Check sheet for the modelled part. Datum: model origin and axes. Units: mm. Face numbers are marked on the shaded views. Round coordinates to 2 decimals unless told otherwise and drop trailing zeros. Order: outer loops, then holes, each group sorted by start corner. A loop starts at its lowest first (then second) coordinate and runs counter-clockwise, first axis right, second up.
(1) Mould release check, pull along X, two halves, no side actions. Record for the marked faces 1, 2, 3 and 4: released by +X, released by -X, zero draft, split by the parting line, or undercut.
(2) Depth check by flat-ended pin: pin 1 (3.5 mm diameter, centred on x = 5, y = 1, fed in from -Z); pin 2 (1.5 mm diameter, centred on x = 44.5, y = -14, fed in from +Z); pin 3 (1 mm diameter, centred on x = -36, z = -36.5, fed in from -Y); pin 4 (3 mm diameter, centred on x = 0, z = -6.25, fed in from +Y). Enter the tip coordinate at first touch or a pass-through.
(3) Sectioned sample at A-A, the plane x = -4. Enter the section's corners in (y, z), and give its area (3 significant figures).
(4) Sectioned sample at C-C, the plane y = -15. Enter the section's corners in (x, z).
(5) Thickness scan on probe 1 along Z at (x, y) = (-7.5, 1.25); probe 2 along X at (y, z) = (0.65, -6.25); probe 3 along Y at (x, z) = (-42.5, -26). Record the ranges inside material, lowest first.
(6) Sectioned sample at B-B, the plane y = -5.25. Enter the section's corners in (x, z), and give its area (3 significant figures).
```python
from build123d import *

# Parameters (mm, degrees)
BOSS_EXTRUDE1_DEPTH             = 2
BOSS_EXTRUDE2_DEPTH             = 17
BOSS_EXTRUDE2_DIRECTION_2_REACH = 86.623
SKETCH7_R                       = 4
CUT_EXTRUDE4_DEPTH              = 117.637747494
FILLET1_R                       = 1
CUT_EXTRUDE1_DEPTH              = 115.868304979
CUT_EXTRUDE2_DEPTH              = 89.209557156
SKETCH5_R                       = 2
CUT_EXTRUDE3_DEPTH              = 89.209557156


with BuildPart() as part:
    # Sketch1 → Boss-Extrude1 (new body)
    with BuildSketch(Plane(origin=(0, 0, 0), x_dir=(1, 0, 0), z_dir=(0, 1, 0))):
        Polygon((25, 46), (-25, 46), (-71, 0), (71, 0), align=None)
    extrude(amount=BOSS_EXTRUDE1_DEPTH)

    # Sketch2 → Boss-Extrude2 (add)
    with BuildSketch(Plane(origin=(0, 0, 0), x_dir=(-1, 0, 0), z_dir=(0, -1, 0))):
        Polygon((25, 46), (71, 0), (72.414213562, 1.414213562), (26.414213562, 47.414213562), align=None)
        Polygon((-26.414213562, 47.414213562), (-72.414213562, 1.414213562), (-71, 0), (-25, 46), align=None)
    extrude(amount=BOSS_EXTRUDE2_DEPTH)

    # Boss-Extrude2 direction 2: up to this face of the body (flat: up to its plane)
    boss_extrude2_direction_2_end = Plane(part.part.faces().sort_by_distance((0, 2, -19.326388889))[0])
    # Sketch2 → Boss-Extrude2 direction 2 (add, up to the picked face)
    with BuildSketch(Plane(origin=(0, 0, 0), x_dir=(-1, 0, 0), z_dir=(0, -1, 0)), mode=Mode.PRIVATE) as boss_extrude2_direction_2_sk1:
        Polygon((25, 46), (71, 0), (72.414213562, 1.414213562), (26.414213562, 47.414213562), align=None)
    boss_extrude2_direction_2_tool1 = split(extrude(boss_extrude2_direction_2_sk1.sketch, amount=-BOSS_EXTRUDE2_DIRECTION_2_REACH, mode=Mode.PRIVATE), bisect_by=boss_extrude2_direction_2_end, keep=Keep.BOTH, mode=Mode.PRIVATE)
    # Sketch2 → Boss-Extrude2 direction 2 (add, up to the picked face)
    with BuildSketch(Plane(origin=(0, 0, 0), x_dir=(-1, 0, 0), z_dir=(0, -1, 0)), mode=Mode.PRIVATE) as boss_extrude2_direction_2_sk2:
        Polygon((-26.414213562, 47.414213562), (-72.414213562, 1.414213562), (-71, 0), (-25, 46), align=None)
    boss_extrude2_direction_2_tool2 = split(extrude(boss_extrude2_direction_2_sk2.sketch, amount=-BOSS_EXTRUDE2_DIRECTION_2_REACH, mode=Mode.PRIVATE), bisect_by=boss_extrude2_direction_2_end, keep=Keep.BOTH, mode=Mode.PRIVATE)
    add(boss_extrude2_direction_2_tool1.solids().sort_by(Axis((-48.707107, 0, -23.707107), (0, 1, 0)))[0])
    add(boss_extrude2_direction_2_tool2.solids().sort_by(Axis((48.707107, 0, -23.707107), (0, 1, 0)))[0])

    # Sketch7 → Cut-Extrude4 (cut, through all)
    with BuildSketch(Plane(origin=(-36.914213562, 0, -36.914213562), x_dir=(-0.7071067811865512, 0, 0.7071067811865438), z_dir=(-0.7071067811865438, 0, -0.7071067811865512))):
        with Locations((38.204581464, -7.5)):
            Circle(SKETCH7_R)
        with Locations((8.204581464, -7.5)):
            Circle(SKETCH7_R)
    cut_extrude4 = extrude(amount=-CUT_EXTRUDE4_DEPTH, mode=Mode.SUBTRACT)

    # Fillet1
    fillet1_edges = [part.edges().sort_by_distance(p)[0] for p in [
        (-49.414213562, 2, -24.414213562),
        (-71.707106781, 2, -0.707106781),
        (71.707106781, 2, -0.707106781),
        (49.414213562, 2, -24.414213562),
        (48, 0, -23),
    ]]
    fillet(fillet1_edges, radius=FILLET1_R)

    # Sketch3 → Cut-Extrude1 (cut, through all)
    with BuildSketch(Plane(origin=(-35.5, 0, -35.5), x_dir=(0.7071067811865511, 0, -0.707106781186544), z_dir=(0.707106781186544, 0, 0.7071067811865511))):
        Polygon((14.849242405, 0), (-2.150757595, -17), (14.849242405, -17), align=None)
    cut_extrude1 = extrude(amount=-CUT_EXTRUDE1_DEPTH, mode=Mode.SUBTRACT)

    # Sketch4 → Cut-Extrude2 (cut, through all)
    with BuildSketch(Plane(origin=(0, 0, 0), x_dir=(-1, 0, 0), z_dir=(0, -1, 0))):
        Polygon((42.943650814, 19.571067812), (29.014718626, 33.5), (0, 33.5), (0, 12.5), (35.872583002, 12.5), align=None)
        Polygon((0, 12.5), (0, 33.5), (-29.014718626, 33.5), (-42.943650814, 19.571067812), (-35.872583002, 12.5), align=None)
    extrude(amount=-CUT_EXTRUDE2_DEPTH, mode=Mode.SUBTRACT)

    # Mirror1: Cut-Extrude4, Cut-Extrude1 across plane
    add(cut_extrude4.mirror(Plane.ZY), mode=Mode.SUBTRACT)
    add(cut_extrude1.mirror(Plane.ZY), mode=Mode.SUBTRACT)

    # Sketch5 → Cut-Extrude3 (cut, through all)
    with BuildSketch(Plane(origin=(0, 0, 0), x_dir=(-1, 0, 0), z_dir=(0, -1, 0))):
        with Locations(Location((0, 6.25, 0), (0, 0, 90))):
            Circle(SKETCH5_R)
        with Locations(Location((0, 39.75, 0), (0, 0, 90))):
            Circle(SKETCH5_R)
        with Locations(Location((-57, 6.25, 0), (0, 0, 90))):
            Circle(SKETCH5_R)
        with Locations(Location((57, 6.25, 0), (0, 0, 270))):
            Circle(SKETCH5_R)
    extrude(amount=-CUT_EXTRUDE3_DEPTH, mode=Mode.SUBTRACT)


solid = part.part
```
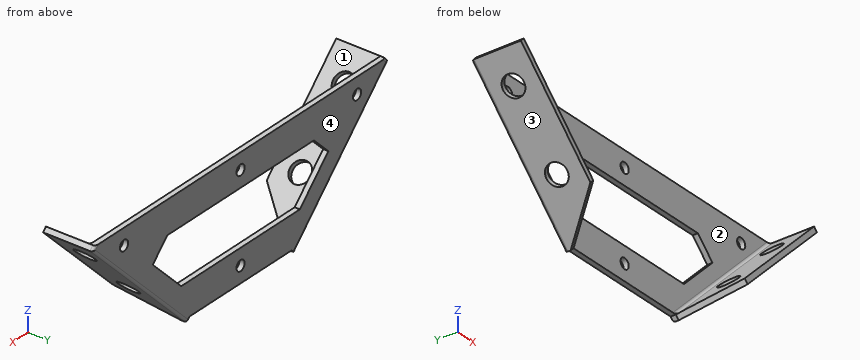
Derived:
1. face 1: undercut
1. face 2: undercut
1. face 3: released by -X
1. face 4: zero draft
2. pin 1: stops at z = -46
2. pin 2: stops at z = -25.75
2. pin 3: stops at y = -15
2. pin 4: passes through
3. outline: (0, -46) - (2, -46) - (2, -33.5) - (0, -33.5) - close; (0, -12.5) - (2, -12.5) - (2, 0) - (0, 0) - close
3. area: 50.0 mm2
4. outline: (-72.41, -1.41) - (-37.02, -36.81) - (-35.61, -35.39) - (-71, 0) - close; (35.61, -35.39) - (37.02, -36.81) - (72.41, -1.41) - (71, 0) - close
5. probe 1: z = -46 to -33.5, -12.5 to 0
5. probe 2: x = -67.58 to -59, -55 to -2, 2 to 55, 59 to 67.58
5. probe 3: y = 0 to 2
6. outline: (-72.41, -1.41) - (-66.27, -7.56) - (-64.85, -6.15) - (-71, 0) - close; (-61.59, -12.24) - (-45.05, -28.77) - (-43.64, -27.36) - (-60.18, -10.82) - close; (-40.38, -33.45) - (-30.13, -43.7) - (-28.71, -42.29) - (-38.96, -32.04) - close; (28.71, -42.29) - (30.13, -43.7) - (40.38, -33.45) - (38.96, -32.04) - close; (43.64, -27.36) - (45.05, -28.77) - (61.59, -12.24) - (60.18, -10.82) - close; (64.85, -6.15) - (66.27, -7.56) - (72.41, -1.41) - (71, 0) - close
6. area: 186 mm2
